Geometry check sheet. Reference: the model listing, model coordinates, mm. A direction names the side the tool comes from. Give positions to 0.01 mm unless a question says otherwise; leave off trailing zeros. Loops run counter-clockwise (first coordinate to the right, second up) from the corner with the lowest first, then second, coordinate; pieces in that order, holes last.
1. Tool access check on faces 4 (the flat face through (15.9, 5, 2)), 5 (the flat face through (16.9, 5, 2)). Record the directions out of +Z, -Z, +X, -X, +Y, -Y that give a thin tool (end or side, any length) a straight path to the whole face; none if there is none.
2. Release check for a two-part mould opening along Y. For faces 1 (the flat face through (12.2, -0.4, 5)), 2 (the flat face through (7, 0, 2)), 3 (the cylindrical face through (16.615, -0.699, 2.535)) record: +Y half, -Y half, draft (parallel to the pull), parting line (faces both ways), or undercut.
3. Cross-section at C-C, the plane x = 11.5. Record the cut outline in (y, z), plus the area to 3 significant figures.
4. Cross-section at A-A, the plane z = 1.9. Record the cut outline in (x, y).
5. Cross-section at B-B, the plane y = 7.5. Record the cut outline in (x, z), plus the area to 3 significant figures.
6. Material ranges on L1, parallel to X at y = 8.5, z = 2.25; L2, parallel to Y at x = 8, z = 0.3; L3, parallel to X at y = -0.25, z = 2.3, recorded low to high.
7. Go/stop test with flat-tipped pins: pin 1 Ø2 at (x, z) = (14.5, 4.5) entering from +Y; pin 2 Ø1 at (x, z) = (4.5, 2) entering from +Y; pin 3 Ø3 at (x, y) = (13, 2) entering from -Z. Record where each tip stops, or that it passes through.
from build123d import *

# Parameters (mm, degrees)
EXTRUDE_THIN1_DEPTH = 5
FILLET1_R           = 1


with BuildPart() as part:
    # Sketch1 → Extrude-Thin1 (new body)
    with BuildSketch(Plane.XY):
        Polygon((0, 0), (15.9, 0), (15.9, 10), (16.9, 10), (16.9, -1), (0, -1), align=None)
    extrude(amount=EXTRUDE_THIN1_DEPTH)

    # Fillet1
    fillet1_edges = [part.edges().sort_by_distance(p)[0] for p in [
        (16.9, -1, 2.5),
        (15.9, 0, 2.5),
    ]]
    fillet(fillet1_edges, radius=FILLET1_R)


solid = part.part
Result:
1. face 4: +Z, -Z, -X, +Y
1. face 5: +Z, -Z, +X, +Y, -Y
2. face 1: draft
2. face 2: +Y half
2. face 3: -Y half
3. outline: (-1, 0) - (0, 0) - (0, 5) - (-1, 5) - close
3. area: 5.00 mm2
4. outline: (0, -1) - (15.9, -1) arc R1 ccw to (16.9, 0) - (16.9, 10) - (15.9, 10) - (15.9, 1) arc R1 cw to (14.9, 0) - (0, 0) - close
5. outline: (15.9, 0) - (16.9, 0) - (16.9, 5) - (15.9, 5) - close
5. area: 5.00 mm2
6. L1: x = 15.9 to 16.9
6. L2: y = -1 to 0
6. L3: x = 0 to 16.87
7. pin 1: stops at y = 0.2
7. pin 2: stops at y = 0
7. pin 3: passes through
